Source: CAD feature listing. Evaluate the final solid. Frame: model axes, mm. Face numbers are marked on the shaded views. A direction names the side the tool comes from. Round coordinates to 2 decimals unless told otherwise and drop trailing zeros. Loops run counter-clockwise (first coordinate to the right, second up) from the corner with the lowest first, then second, coordinate; pieces in that order, holes last. Notation, with made-up numbers: (65, -10.5) -> (117, -10.5) arc R6 ccw to (117, 0.5) -> close; hole circle Ø9 at (-34, 84). An arc over 180 degrees is marked (long way). Return JSON: item names as keys, results as strings. Group by question number.
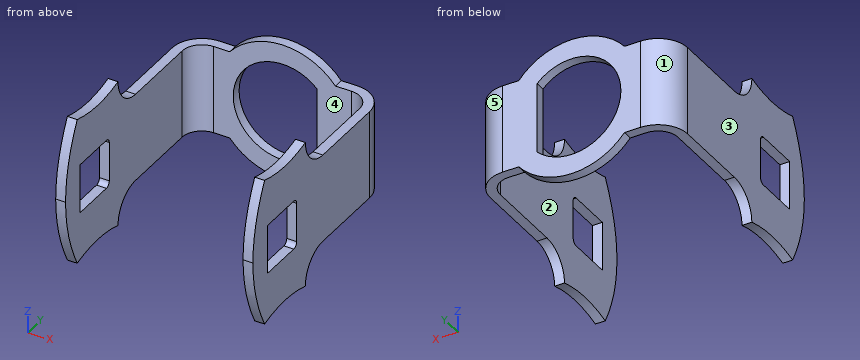
```python
from build123d import *

# Parameters (mm, degrees)
BOSS_EXTRUDE1_DEPTH = 15
CUT_EXTRUDE2_DEPTH  = 34.970575503
CUT_EXTRUDE3_DEPTH  = 14
CUT_EXTRUDE4_DEPTH  = 34.970575503
CUT_EXTRUDE5_DEPTH  = 34.970575606
FILLET1_R           = 3
FILLET2_R           = 3
SKETCH7_W           = 5
SKETCH7_H           = 5
CUT_EXTRUDE6_DEPTH  = 34.970575606
FILLET3_R           = 0.5


with BuildPart() as part:
    # Sketch1 → Boss-Extrude1 (new body)
    with BuildSketch(Plane.XY):
        with BuildLine():
            Line((-19, 0), (-19, 20))
            ThreePointArc((-19, 20), (-18.414213562, 21.414213562), (-17, 22))
            Line((-17, 22), (-3, 22))
            ThreePointArc((-3, 22), (-1.585786438, 21.414213562), (-1, 20))
            Line((-1, 20), (-1, 0))
            Line((-1, 0), (0, 0))
            Line((0, 0), (0, 20))
            ThreePointArc((0, 20), (-0.878679656, 22.121320344), (-3, 23))
            Line((-3, 23), (-17, 23))
            ThreePointArc((-17, 23), (-19.121320344, 22.121320344), (-20, 20))
            Line((-20, 20), (-20, 0))
            Line((-20, 0), (-19, 0))
        make_face()
    extrude(amount=BOSS_EXTRUDE1_DEPTH)

    # Sketch2 → Cut-Extrude2 (cut, through all)
    with BuildSketch(Plane(origin=(0, 23, 0), x_dir=(1, 0, 0), z_dir=(0, 1, 0))):
        with BuildLine():
            Line((-6.5, -11.070714214), (-6.5, -3.929285786))
            ThreePointArc((-6.5, -3.929285786), (-15, -7.5), (-6.5, -11.070714214))
        make_face()
    extrude(amount=-CUT_EXTRUDE2_DEPTH, mode=Mode.SUBTRACT)

    # Sketch4 → Cut-Extrude3 (cut)
    with BuildSketch(Plane(origin=(0, 23, 0), x_dir=(1, 0, 0), z_dir=(0, 1, 0))):
        with BuildLine():
            Line((-4.638097353, -12), (0, -12))
            Line((0, -12), (0, -15))
            Line((0, -15), (-20, -15))
            Line((-20, -15), (-20, -12))
            Line((-20, -12), (-15.361902647, -12))
            ThreePointArc((-15.361902647, -12), (-10, -14.5), (-4.638097353, -12))
        make_face()
        with BuildLine():
            Line((-4.638097353, -3), (0, -3))
            Line((0, -3), (0, 0))
            Line((0, 0), (-20, 0))
            Line((-20, 0), (-20, -3))
            Line((-20, -3), (-15.361902647, -3))
            ThreePointArc((-15.361902647, -3), (-10, -0.5), (-4.638097353, -3))
        make_face()
    extrude(amount=-CUT_EXTRUDE3_DEPTH, mode=Mode.SUBTRACT)

    # Sketch5 → Cut-Extrude4 (cut, through all)
    with BuildSketch(Plane.ZY.offset(20)):
        with BuildLine():
            Line((0, 2), (0, 0))
            Line((0, 0), (7.5, 0))
            add(Edge.make_bspline(
                [(0, 2), (3.75, 0), (7.5, 0)],
                knots=[0, 0, 0, 0.5, 0.5, 0.5], degree=2))
        make_face()
        with BuildLine():
            add(Edge.make_bspline(
                [(7.5, 0), (11.25, 0), (15, 2)],
                knots=[0.5, 0.5, 0.5, 1, 1, 1], degree=2))
            Line((7.5, 0), (15, 0))
            Line((15, 0), (15, 2))
        make_face()
    extrude(amount=-CUT_EXTRUDE4_DEPTH, mode=Mode.SUBTRACT)

    # Sketch6 → Cut-Extrude5 (cut, through all)
    with BuildSketch(Plane.ZY.offset(20)):
        with BuildLine():
            Line((0, 9), (0, 5.5))
            Line((0, 5.5), (0.5, 5.5))
            add(Edge.make_bspline(
                [(0, 9), (0.5, 7.25), (0.5, 5.5)],
                knots=[0, 0, 0, 0.5, 0.5, 0.5], degree=2))
        make_face()
        with BuildLine():
            Line((0.5, 5.5), (0, 5.5))
            Line((0, 5.5), (0, 2))
            add(Edge.make_bspline(
                [(0.5, 5.5), (0.5, 3.75), (0, 2)],
                knots=[0.5, 0.5, 0.5, 1, 1, 1], degree=2))
        make_face()
        with BuildLine():
            Line((15, 9), (15, 2))
            add(Edge.make_bspline(
                [(15, 9), (14, 5.5), (15, 2)],
                knots=[0, 0, 0, 1, 1, 1], degree=2))
        make_face()
    extrude(amount=-CUT_EXTRUDE5_DEPTH, mode=Mode.SUBTRACT)

    # Fillet1
    fillet1_edges = [part.edges().sort_by_distance(p)[0] for p in [
        (-19.5, 9, 3),
    ]]
    fillet(fillet1_edges, radius=FILLET1_R - 0.0001)  # a hair under: the kernel refuses the full size

    # Fillet2
    fillet2_edges = [part.edges().sort_by_distance(p)[0] for p in [
        (-0.5, 9, 3),
        (-0.5, 9, 12),
        (-19.5, 9, 12),
    ]]
    fillet(fillet2_edges, radius=FILLET2_R - 0.0001)  # a hair under: the kernel refuses the full size

    # Sketch7 → Cut-Extrude6 (cut, through all)
    with BuildSketch(Plane.ZY.offset(20)):
        with Locations((7.5, 5)):
            Rectangle(SKETCH7_W, SKETCH7_H)
    extrude(amount=-CUT_EXTRUDE6_DEPTH, mode=Mode.SUBTRACT)

    # Fillet3
    fillet3_edges = [part.edges().sort_by_distance(p)[0] for p in [
        (-0.5, 7.5, 5),
        (-19.5, 7.5, 5),
        (-0.5, 7.5, 10),
        (-19.5, 7.5, 10),
    ]]
    fillet(fillet3_edges, radius=FILLET3_R)


solid = part.part
```
(1) Mould query, pull axis X, two halves, no side actions, for the marked faces 3, 4 and 5. Classes: released by +X, released by -X, zero draft, split by the parting line, or undercut.
(2) Cut plane A-A (x = -10). Return loops of the section in (y, z).
(3) Set-up query: the marked faces 1 and 2. Return all of +Z, -Z, +X, -X, +Y, -Y with unobstructed straight access to the full face (end or side cutting, diameter ignored); none if empty.
(4) Cut plane B-B (y = 10.5). Return loops of the section in (x, z).
(5) Ray query, line 1 (Z direction, x = -10, y = 22.5); line 2 (X direction, y = 10.75, z = 11.25); line 3 (Y direction, x = -7.5, z = 1). Return the intervals inside material, ascending.
(6) Pin query (flat end, axial travel): pin 1 (0.8 mm diameter, centred on x = -19.5, y = 4.5, fed in from +Z); pin 2 (4.5 mm diameter, centred on y = 7, z = 7.5, fed in from -X); pin 3 (0.5 mm diameter, centred on x = -19.5, z = 8, fed in from -Y); pin 4 (0.5 mm diameter, centred on x = -0.5, y = 4.5, fed in from -Z). Return the tip coordinate at first contact, or that it passes through.
(7) Cut plane C-C (z = 13.5). Count the separate pieces of the cut face and the enclosed holes in it, and give its area (3 significant figures).
Answers follow:
{
 "1": {"face 3": "released by -X", "face 4": "undercut", "face 5": "released by +X"},
 "2": {"outline": "(22, 0.5) -> (23, 0.5) -> (23, 2.5) -> (22, 2.5) -> close; (22, 12.5) -> (23, 12.5) -> (23, 14.5) -> (22, 14.5) -> close"},
 "3": {"face 1": "+Z, -Z, -X, +Y", "face 2": "+Z, -Z, -Y"},
 "4": {"outline": "(-20, 2.6) -> (-19, 2.6) -> (-19, 12.4) -> (-20, 12.4) -> close; (-1, 2.6) -> (0, 2.6) -> (0, 12.4) -> (-1, 12.4) -> close"},
 "5": {"line 1": "0.5 to 2.5, 12.5 to 14.5", "line 2": "-20 to -19, -1 to 0", "line 3": "22 to 23"},
 "6": {"pin 1": "z = 14.58", "pin 2": "x = -20", "pin 3": "y = 0", "pin 4": "z = 0.44"},
 "7": {"separate pieces": "3", "enclosed holes": "0", "area": "23.5 mm^2"}
}
